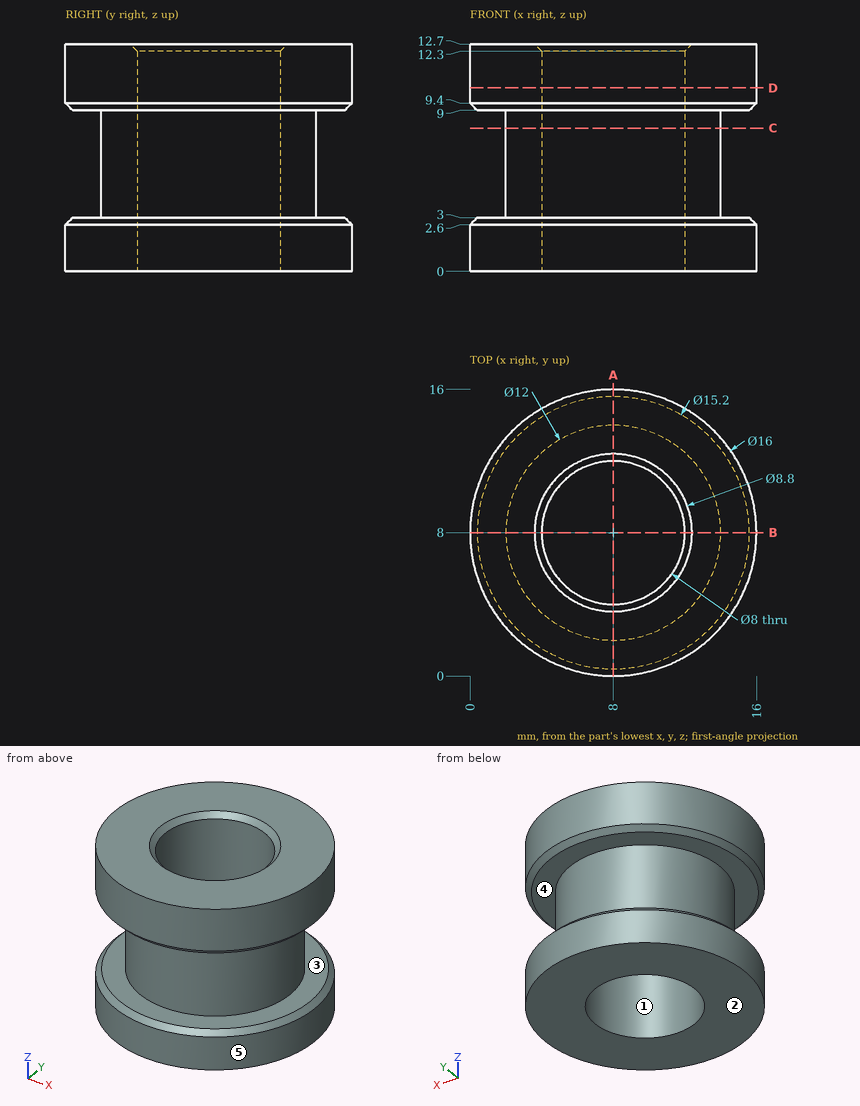
Part print with two shaded views. Sizes in mm from the minimum x, y, z corner. A direction names the side the tool comes from. Coordinates: 2 decimals unless noted, no trailing zeros. Write each loop counter-clockwise with the first axis right and the second up, starting at its lowest first coordinate (ties: lowest second). Pieces come first, ordered by that corner, then holes.
(1) Cut at C-C on z = 8. List the corners of the cut face in (x, y), and give its area (3 significant figures).
(2) Cut at D-D on z = 10.25. List the corners of the cut face in (x, y).
(3) Mould opens along Z. For the marked faces 1, 2 and 3 say: pulls with the +Z half, pulls with the -Z half, needs draft (parallel to the pull), parting line crosses it, or undercut.
(4) 3-axis set-ups, long thin cutter, end or side, ignore diameter. For the marked faces 4 and 5: which of +Z, -Z, +X, -X, +Y, -Y reach the whole face in a straight line?
(5) Drill centre lines: line 1 (Z direction, x = 2.75, y = 3); line 2 (Y direction, x = 8, z = 4); line 3 (Y direction, x = 7.25, z = 5). Where is each one in solid material? Low to high.
(6) Cut at A-A on x = 8. List the corners of the cut face in (y, z), and give its area (3 significant figures).
(7) Pin check, flat tips, straight feed: pin 1 Ø7.5 at (x, y) = (9.5, 9.5) entering from +Z; pin 2 Ø4 at (y, z) = (5, 11) entering from -X; pin 3 Ø1 at (y, z) = (13, 8) entering from +X; pin 4 Ø1.5 at (y, z) = (5.5, 5.5) entering from +X. Stop position of each tip, or through.
Working result:
1. outline: circle Ø12 at (8, 8); hole circle Ø8 at (8, 8)
1. area: 62.8 mm2
2. outline: circle Ø16 at (8, 8); hole circle Ø8 at (8, 8)
3. face 1: needs draft
3. face 2: pulls with the -Z half
3. face 3: undercut
4. face 4: none
4. face 5: +Z, -Z
5. line 1: z = 0 to 3, 9 to 12.7
5. line 2: y = 2 to 4, 12 to 14
5. line 3: y = 2.05 to 4.07, 11.93 to 13.95
6. outline: (0, 0) - (4, 0) - (4, 12.3) - (3.6, 12.7) - (0, 12.7) - (0, 9.4) - (0.4, 9) - (2, 9) - (2, 3) - (0.4, 3) - (0, 2.6) - close; (12, 0) - (16, 0) - (16, 2.6) - (15.6, 3) - (14, 3) - (14, 9) - (15.6, 9) - (16, 9.4) - (16, 12.7) - (12.4, 12.7) - (12, 12.3) - close
6. area: 77.1 mm2
7. pin 1: stops at z = 12.7
7. pin 2: stops at x = 0.06
7. pin 3: stops at x = 11.97
7. pin 4: stops at x = 13.74
